from build123d import *

# Parameters (mm, degrees)
F0_R      = 152.4
F0_R_2    = 127
F1_DEPTH  = 101.6
F2_R      = 127.018603898
F3_DEPTH  = 25.4
F5_R      = 6.35
F6_DEPTH  = 304.801
F9_R      = 152.4
F7_R      = 76.2
F13_DEPTH = 25.4
F15_DEPTH = 25.4


with BuildPart() as f1:
    # F0 (on Top) → F1 (new body)
    with BuildSketch(Plane.XY):
        Circle(F0_R)
        Circle(F0_R_2, mode=Mode.SUBTRACT)
    extrude(amount=F1_DEPTH)

    # F2 (on face) → F3 (join)
    with BuildSketch(Plane(origin=(0, 0, 0), x_dir=(1, 0, 0), z_dir=(0, 0, -1))):
        Circle(F2_R)
    extrude(amount=-F3_DEPTH)

    # F5 (on offset) → F6 (cut, through all)
    with BuildSketch(Plane.XZ.offset(152.4)):
        with Locations((0, 50.8)):
            Circle(F5_R)
    extrude(amount=-F6_DEPTH, mode=Mode.SUBTRACT)

    # F9 (on offset) → F10 section 0
    with BuildSketch(Plane(origin=(0, 0, -152.4), x_dir=(1, 0, 0), z_dir=(0, 0, -1))):
        Circle(F9_R)
    # F7 (on face) → F10 section 1
    with BuildSketch(Plane(origin=(0, 0, 0), x_dir=(1, 0, 0), z_dir=(0, 0, -1))):
        Circle(F7_R)
    loft()

    # F12 (on Front) → F13 (join, symmetric)
    with BuildSketch(Plane.XZ):
        Polygon((-177.8, -152.4), (-265.7881810245, -304.8), (-207.1293936748, -304.8), (-148.4706063252, -203.2), (-54.7293936748, -203.2), (-25.4, -152.4), align=None)
        Polygon((148.4706063252, -203.2), (207.1293936748, -304.8), (265.7881810245, -304.8), (177.8, -152.4), (25.4, -152.4), (54.7293936748, -203.2), align=None)
    extrude(amount=F13_DEPTH, both=True)

    # F14 (on Right) → F15 (join, symmetric)
    with BuildSketch(Plane.YZ):
        Polygon((-25.4, -152.4), (-177.8, -152.4), (-265.7881810245, -304.8), (-207.1293936748, -304.8), (-148.4706063252, -203.2), (-54.7293936748, -203.2), align=None)
        Polygon((265.7881810245, -304.8), (177.8, -152.4), (25.4, -152.4), (54.7293936748, -203.2), (148.4706063252, -203.2), (207.1293936748, -304.8), align=None)
    extrude(amount=F15_DEPTH, both=True)


solid = f1.part
Geometry: final body of the model. Coordinates: model frame, mm. A direction names the side the tool comes from. Give positions to 0.01 mm unless a question says otherwise; leave off trailing zeros. Write each loop counter-clockwise with the first axis right and the second up, starting at its lowest first coordinate (ties: lowest second). Pieces come first, ordered by that corner, then holes.
(1) Cut plane A-A, the plane z = -180. Return loops of the section in (x, y).
(2) Ray query, line 1 (Z direction, x = 0, y = 141); line 2 (Y direction, x = -149.5, z = -164); line 3 (Z direction, x = 0, y = -142). Return the intervals inside material, ascending.
(3) Access query for faces 5 (the flat face through (101, 0, -203.2)), 6 (the flat face through (73, -75, -152.4)), 7 (the flat face through (-2, -2, 25.4)), 8 (the flat face through (0, 101, -203.2)). Directions: +Z, -Z, +X, -X, +Y, -Y. A direction counts if a zero-diameter tool reaches every point of the face in a straight line with its end or side. Return the directions, or none.
(4) Cut plane D-D, the plane z = -94.5. Return loops of the section in (x, y), then the cut area to 3 significant figures.
(5) Mould query, pull axis Z, two halves, no side actions, for faces 1 (the flat face through (-147, -25.4, -194)), 2 (the flat face through (-0.356, -40.27, -178.156)), 3 (the flat face through (32, 70, 0)), 4 (the conical face through (-19.156, 86.265, -24.333)). Classes: released by +Z, released by -Z, zero draft, split by the parting line, or undercut.
(6) Cut plane C-C, the plane y = 228.5. Return loops of the section in (x, z), then the cut area to 3 significant figures.
(7) Cut plane B-B, the plane z = -31.5. Return loops of the section in (x, y), then the cut area to 3 significant figures.
(8) First-contact query: P1, Ø8, axis at x = 66, y = -28.5, coming from the -Z side; P2, Ø1, axis at y = -42, z = -114, coming from the -X side; P3, Ø1, axis at y = -31.5, z = -154, coming from the +X side. Flat tips, straight axial feed; report the tip coordinate or a pass-through.
Values follow:
1. outline: (-193.73, -25.4) - (-41.33, -25.4) - (-41.33, 25.4) - (-193.73, 25.4) - close; (-25.4, -193.73) - (25.4, -193.73) - (25.4, -41.33) - (-25.4, -41.33) - close; (-25.4, 41.33) - (25.4, 41.33) - (25.4, 193.73) - (-25.4, 193.73) - close; (41.33, -25.4) - (193.73, -25.4) - (193.73, 25.4) - (41.33, 25.4) - close
2. line 1: z = -203.2 to -129.6, 0 to 44.45, 57.15 to 101.6
2. line 2: y = -25.4 to 25.4
2. line 3: z = -203.2 to -131.6, 0 to 44.45, 57.15 to 101.6
3. face 5: -Z, +Y, -Y
3. face 6: -Z, +X, -Y
3. face 7: +Z
3. face 8: -Z, +X, -X
4. outline: circle Ø246.9 at (0, 0)
4. area: 47,900 mm2
5. face 1: zero draft
5. face 2: released by -Z
5. face 3: undercut
5. face 4: undercut
6. outline: (-25.4, -304.8) - (25.4, -304.8) - (25.4, -240.21) - (-25.4, -240.21) - close
6. area: 3,280 mm2
7. outline: circle Ø183.9 at (0, 0)
7. area: 26,600 mm2
8. P1: stops at z = -203.2
8. P2: stops at x = -126.72
8. P3: stops at x = 25.4
